The figure shows three views and two pictorial views of one solid part (mm, origin at its lowest corner). Answer the questions. A direction names the side the tool comes from. Coordinates: 2 decimals unless noted, no trailing zeros. Order: outer loops, then holes, each group sorted by start corner. A loop starts at its lowest first (then second) coordinate and runs counter-clockwise, first axis right, second up. Notation, with made-up numbers: M 50,-30.75 L 105,-30.75 A8 cw 105,-17.75 Z; hole C 62.5,43.5 d2. An arc over 180 degrees is marked long. Write item = value, one per line. Start each with the question number.
Q1. Find section B-B on y = 15.2. Give the vertices of the cut face in (x, z).
Q2. Straight lines are drawn through the part: line 1 along Y through (x, z) = (6, 4.4); line 2 along X through (y, z) = (33.7, 1.05); line 3 along Y through (x, z) = (15.2, 3.9). For each, find the intervals that lie inside material, in ascending order.
Q3. Each of these flat-tipped pins is pushed along its axis until it touches: P1, Ø3, axis at x = 6.2, y = 4.7, coming from the -Z side; P2, Ø1.5, axis at x = 18, z = 4.5, coming from the +Y side; P3, Ø2.5, axis at y = 15.5, z = 2.5, coming from the +X side. Where does it stop, or does it pass through?
Q4. Find section C-C on z = 1. Give the vertices of the cut face in (x, y).
Q5. Determine the mould class of the marked faces 4, 5, 6 and 7 for opening direction Y: released by +Y, released by -Y, zero draft, split by the parting line, or undercut.
Q6. A tool of negligible diameter and unlimited length cuts with its end or side. For the marked faces 1, 2 and 3, from which of +Z, -Z, +X, -X, +Y, -Y can it reach the whole face along a straight path? Write none if from no direction.
Q7. Find section A-A on x = 15.2. Give the vertices of the cut face in (y, z), and give its area (3 significant figures).
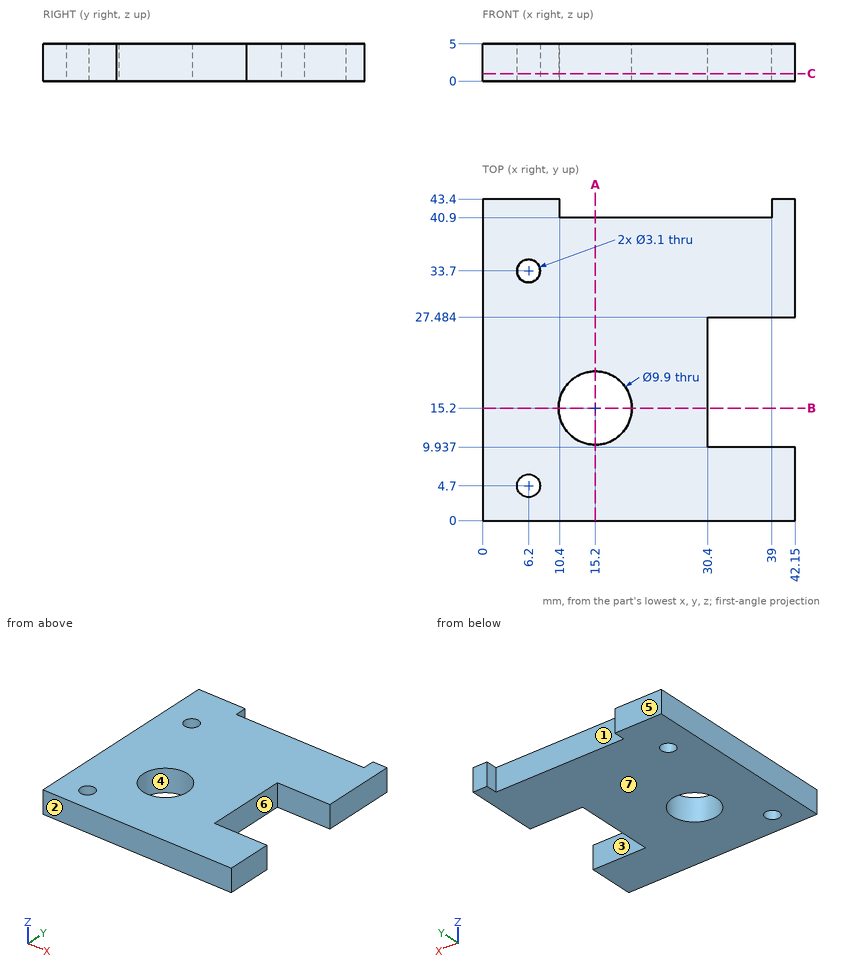
Findings below:
q1.outline = M 0,0 L 10.25,0 L 10.25,5 L 0,5 Z; M 20.15,0 L 30.4,0 L 30.4,5 L 20.15,5 Z
q2.line_1 = 0 to 3.16, 6.24 to 32.16, 35.24 to 43.4
q2.line_2 = 0 to 4.65, 7.75 to 42.15
q2.line_3 = 0 to 10.25, 20.15 to 40.9
q3.P1 = through
q3.P2 = 40.9
q3.P3 = 30.4
q4.outline = M 0,0 L 42.15,0 L 42.15,9.94 L 30.4,9.94 L 30.4,27.48 L 42.15,27.48 L 42.15,43.4 L 39,43.4 L 39,40.9 L 10.4,40.9 L 10.4,43.4 L 0,43.4 Z; hole C 6.2,4.7 d3.1; hole C 6.2,33.7 d3.1; hole C 15.2,15.2 d9.9
q5.face_4 = undercut
q5.face_5 = released by +Y
q5.face_6 = undercut
q5.face_7 = zero draft
q6.face_1 = +Z, -Z, +Y
q6.face_2 = +Z, -Z, +X, -X, -Y
q6.face_3 = +Z, -Z, +X
q7.outline = M 0,0 L 10.25,0 L 10.25,5 L 0,5 Z; M 20.15,0 L 40.9,0 L 40.9,5 L 20.15,5 Z
q7.area = 155 mm^2
